Read the model definition and answer for the solid it produces. Units are mm, in the model's axes. A direction names the side the tool comes from. Give positions to 0.01 mm unless a question says otherwise; leave off trailing zeros. Order: outer loops, then holes, each group sorted by start corner. A loop starts at its lowest first (then second) coordinate and runs counter-clockwise, first axis right, second up. Notation, with made-up numbers: (82, 20) -> (93, 20) arc R31 cw to (93, 48) -> close; hole circle Ø3 at (16, 79.25). An arc over 180 degrees is marked (long way). Answer as CSV lines item,"result". Start each with the question number.
1) The mould has two halves that part along Y. Classify faces 3 (the face through (2, 26.67, 2)), 4 (the face through (0, 34.29, 0)), 5 (the face through (1.323, 30.462, -10.074)): +Y half, -Y half, draft (parallel to the pull), parting line (faces both ways), or undercut.
2) Flat-ended cylindrical pins translate along their axes: pin 1 Ø8 at (y, z) = (26.5, -6) entering from +X; pin 2 Ø12 at (x, z) = (-8, 7.5) entering from -Y; pin 3 Ø3 at (y, z) = (13.5, 0.5) entering from +X. Find the tip coordinate at first contact, or state that the pin passes through.
3) Find section A-A (z = 0). Determine the outline of the cut face in (x, y).
4) Straight lines are drawn through the part: L1, parallel to Y at x = 4, z = -3.75; L2, parallel to Y at x = -8.75, z = -1.5; L3, parallel to Z at x = 1.5, y = -18. For each, find the intervals that lie inside material, in ascending order. Write a range as from..to.
5) Find section C-C (y = 16.5). Determine the outline of the cut face in (x, z).
6) For faces 1 (the face through (0, -34.29, 0)), 2 (the face through (-2, -26.67, 2)), determine the directions among +Z, -Z, +X, -X, +Y, -Y from which every point of the face is accessible in a straight line to the end or side of a thin tool.
7) Find section B-B (x = 0). Determine the outline of the cut face in (y, z).
Autodesk Fusion 360 part; units mm, degrees
sketch "Sketch1" plane through (0, 0, 0) normal (0, 1, 0) x (1, 0, 0)
  circle A0 centre (0, 0) radius 2.54
  dimension "d1" = 5.08
extrude "Extrude1" add sketch "Sketch1" along normal mid plane 53.34
sketch "Sketch2" plane through (0, -26.67, 0) normal (0, -1, 0) x (1, 0, 0)
  circle A0 centre (0, 0) radius 2.54
  circle A1 centre (0, 0) radius 10.16
  dimension "d8" = 20.32
extrude "Extrude2" add sketch "Sketch2" along normal blind 7.62 contours A0 | A1
sketch "Sketch3" plane through (0, 26.67, 0) normal (0, 1, 0) x (-1, 0, 0)
  circle A0 centre (0, 0) radius 2.54
  circle A1 centre (0, 0) radius 10.16
  dimension "d9" = 20.32
extrude "Extrude3" add sketch "Sketch3" along normal blind 7.62 contours A0 | A1
fillet "Fillet1" radius 2.54 3 edges at (-9.4724, -34.29, -3.674) (9.4724, 34.29, -3.674) (-9.4724, -26.67, -3.674) 1 faces at (-10.1474, 29.21, -0.5064)
Findings below:
1,face 3,"undercut"
1,face 4,"+Y half"
1,face 5,"draft"
2,pin 1,"x = 9.75"
2,pin 2,"y = -34.29"
2,pin 3,"x = 2.54"
3,outline,"(-10.16, -31.75) arc R2.54 ccw to (-7.62, -34.29) -> (7.62, -34.29) arc R2.54 ccw to (10.16, -31.75) -> (10.16, -29.21) arc R2.54 ccw to (7.62, -26.67) -> (2.54, -26.67) -> (2.54, 26.67) -> (7.62, 26.67) arc R2.54 ccw to (10.16, 29.21) -> (10.16, 31.75) arc R2.54 ccw to (7.62, 34.29) -> (-7.62, 34.29) arc R2.54 ccw to (-10.16, 31.75) -> (-10.16, 29.21) arc R2.54 ccw to (-7.62, 26.67) -> (-2.54, 26.67) -> (-2.54, -26.67) -> (-7.62, -26.67) arc R2.54 ccw to (-10.16, -29.21) -> close"
4,L1,"-34.29..-26.67, 26.67..34.29"
4,L2,"-33.96..-27, 27..33.96"
4,L3,"-2.05..2.05"
5,outline,"circle Ø5.08 at (0, 0)"
6,face 1,"+Z, -Z, +X, -X, -Y"
6,face 2,"none"
7,outline,"(-34.29, -7.62) arc R2.54 ccw to (-31.75, -10.16) -> (-29.21, -10.16) arc R2.54 ccw to (-26.67, -7.62) -> (-26.67, -2.54) -> (26.67, -2.54) -> (26.67, -7.62) arc R2.54 ccw to (29.21, -10.16) -> (31.75, -10.16) arc R2.54 ccw to (34.29, -7.62) -> (34.29, 7.62) arc R2.54 ccw to (31.75, 10.16) -> (29.21, 10.16) arc R2.54 ccw to (26.67, 7.62) -> (26.67, 2.54) -> (-26.67, 2.54) -> (-26.67, 7.62) arc R2.54 ccw to (-29.21, 10.16) -> (-31.75, 10.16) arc R2.54 ccw to (-34.29, 7.62) -> close"
